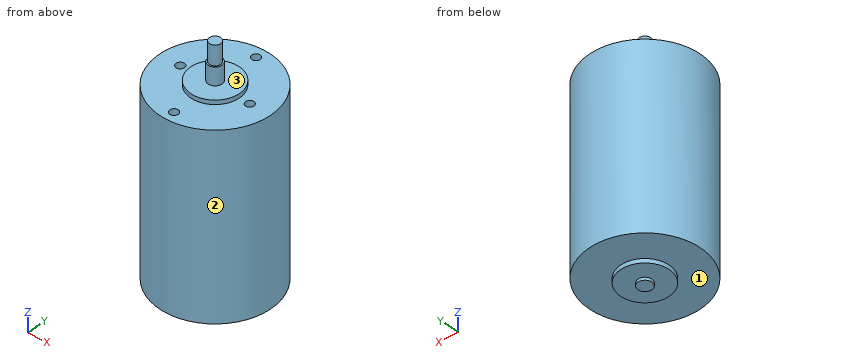
from build123d import *

# Parameters (mm, degrees)
SKETCH_3_R          = 20
EXTRUDE_1_DEPTH     = 65
SKETCH_4_R          = 8.75
EXTRUDE_2_DEPTH     = 1.5
SKETCH_6_R          = 8.75
EXTRUDE_3_DEPTH     = 1.5
SKETCH_7_R          = 2.5
EXTRUDE_4_DEPTH     = 6.3
SKETCH_8_R          = 2
EXTRUDE_5_DEPTH     = 7
SKETCH_10_R         = 2.5
EXTRUDE_6_DEPTH     = 1
SKETCH_11_R         = 1.5
CUT_EXTRUDE_1_DEPTH = 4
SKETCH_12_R         = 1.5
CUT_EXTRUDE_2_DEPTH = 4


with BuildPart() as part:
    # 草圖3 → 填料-伸長1 (new body)
    with BuildSketch(Plane.XY):
        Circle(SKETCH_3_R)
    extrude(amount=EXTRUDE_1_DEPTH)

    # 草圖4 → 填料-伸長2 (add)
    with BuildSketch(Plane(origin=(0, 0, 0), x_dir=(-1, 0, 0), z_dir=(0, 0, -1))):
        Circle(SKETCH_4_R)
    extrude(amount=EXTRUDE_2_DEPTH)

    # 草圖6 → 填料-伸長3 (add)
    with BuildSketch(Plane.XY.offset(65)):
        Circle(SKETCH_6_R)
    extrude(amount=EXTRUDE_3_DEPTH)

    # 草圖7 → 填料-伸長4 (add)
    with BuildSketch(Plane.XY.offset(66.5)):
        Circle(SKETCH_7_R)
    extrude(amount=EXTRUDE_4_DEPTH)

    # 草圖8 → 填料-伸長5 (add)
    with BuildSketch(Plane.XY.offset(72.8)):
        Circle(SKETCH_8_R)
    extrude(amount=EXTRUDE_5_DEPTH)

    # 草圖10 → 填料-伸長6 (add)
    with BuildSketch(Plane(origin=(0, 0, -1.5), x_dir=(-1, 0, 0), z_dir=(0, 0, -1))):
        Circle(SKETCH_10_R)
    extrude(amount=EXTRUDE_6_DEPTH)

    # 草圖11 → 除料-伸長1 (cut)
    with BuildSketch(Plane.XY.offset(65)):
        with Locations((-12.5, 0)):
            Circle(SKETCH_11_R)
        with Locations((12.5, 0)):
            Circle(SKETCH_11_R)
    extrude(amount=-CUT_EXTRUDE_1_DEPTH, mode=Mode.SUBTRACT)

    # 草圖12 → 除料-伸長2 (cut)
    with BuildSketch(Plane.XY.offset(65)):
        with Locations((0, 16.25)):
            Circle(SKETCH_12_R)
        with Locations((0, -16.25)):
            Circle(SKETCH_12_R)
    extrude(amount=-CUT_EXTRUDE_2_DEPTH, mode=Mode.SUBTRACT)


solid = part.part
Geometry check sheet. Reference: the model listing, model coordinates, mm. Face numbers are marked on the shaded views. A direction names the side the tool comes from. Give positions to 0.01 mm unless a question says otherwise; leave off trailing zeros. Order: outer loops, then holes, each group sorted by start corner. A loop starts at its lowest first (then second) coordinate and runs counter-clockwise, first axis right, second up.
1. Sectioned sample at C-C (z = 17). Record the boundary of the cut face in (x, y), then the cut area to 3 significant figures.
Completed:
outline: circle Ø40 at (0, 0)
area: 1,260 mm2
2. Depth check by flat-ended pin: pin 1 (3.5 mm diameter, centred on x = 0.5, y = 16.5, fed in from +Z); pin 2 (10 mm diameter, centred on x = -6.5, z = 37, fed in from +Y); pin 3 (2.5 mm diameter, centred on x = 12.5, y = 0, fed in from +Z). Enter the tip coordinate at first touch or a pass-through.
Completed:
pin 1: stops at z = 65
pin 2: stops at y = 19.94
pin 3: stops at z = 61
3. Sectioned sample at D-D (x = 7.5). Record the boundary of the cut face in (y, z), then the cut area to 3 significant figures.
Completed:
outline: (-18.54, 0) - (-4.51, 0) - (-4.51, -1.5) - (4.51, -1.5) - (4.51, 0) - (18.54, 0) - (18.54, 65) - (4.51, 65) - (4.51, 66.5) - (-4.51, 66.5) - (-4.51, 65) - (-18.54, 65) - close
area: 2,440 mm2
4. Access from +Z, -Z, +X, -X, +Y, -Y to the whole of each face (thin tool, end or side, straight path). Record for the marked faces 1, 2 and 3.
Completed:
face 1: -Z
face 2: +Z, -Z
face 3: +Z
5. Scan lines: line 1 (Y direction, x = 0, z = 63.6); line 2 (Z direction, x = 12, y = 12.5); line 3 (Z direction, x = 5.5, y = -1). Record each from-to range of solid material in increasing order.
Completed:
line 1: y = -20 to -17.75, -14.75 to 14.75, 17.75 to 20
line 2: z = 0 to 65
line 3: z = -1.5 to 66.5
